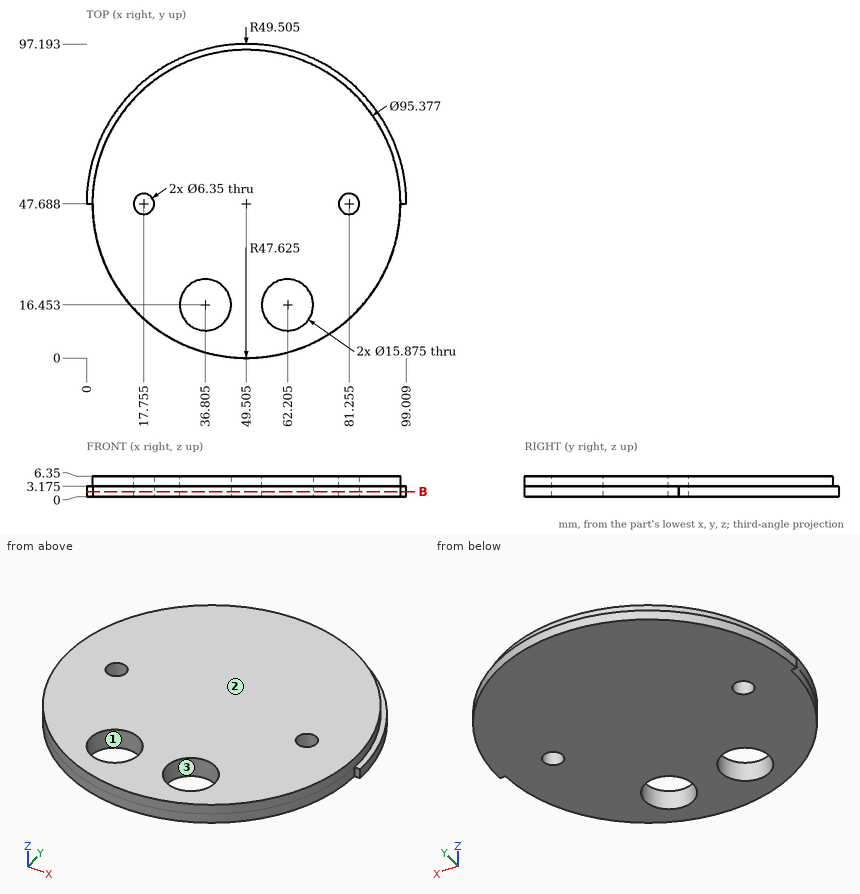
Geometry: see drawing. Coordinates: mm, zero at the bounding-box minimum. Coordinates: 2 decimals unless noted, no trailing zeros. Write each question's results on one line, items separated by ' | '. Start each with the question number.
1) Material intervals for line 1 along X through (y, z) = (20, 1.75) (1 decimal); line 2 along X through (y, z) = (19, 6.25) (1 decimal); line 3 along Y through (x, z) = (58, 1.5) (1 decimal), sorted ascending.
2) Mould query, pull axis X, two halves, no side actions, for the marked faces 1, 2 and 3. Classes: released by +X, released by -X, zero draft, split by the parting line, or undercut.
3) First-contact query: pin 1 (0.6 mm diameter, centred on x = 98, z = 2, fed in from -Y); pin 2 (12.5 mm diameter, centred on x = 36.8, y = 16.45, fed in from +Z); pin 3 (1.5 mm diameter, centred on x = 22, z = 1.5, fed in from -Y); pin 4 (1.5 mm diameter, centred on x = 25.5, z = 4.5, fed in from -Y) (1 decimal). Flat tips, straight axial feed; report the tip coordinate or a pass-through.
4) Cut plane B-B, the plane z = 1.5. State how many separate pieces and enclosed holes the cut face has, and give its area (3 significant figures).
Checks:
1) line 1: 10.8 to 29.7, 43.9 to 55.1, 69.3 to 88.3 | line 2: 11.4 to 29.3, 44.3 to 54.7, 69.7 to 87.6 | line 3: 0.8 to 9.7, 23.2 to 96.5
2) face 1: undercut | face 2: zero draft | face 3: undercut
3) pin 1: y = 47.69 | pin 2: through | pin 3: y = 8.29 | pin 4: y = 6.1
4) separate pieces: 1 | enclosed holes: 4 | area: 6,950 mm^2
